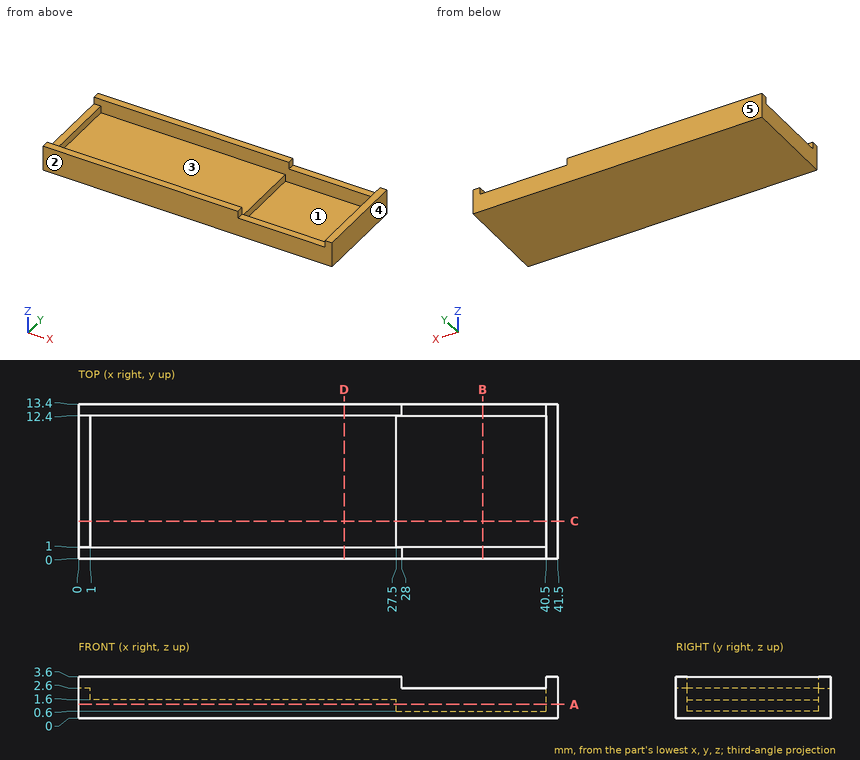
Input: dimensioned drawing with shaded views. Units: mm. Origin: part minimum x, y, z. A direction names the side the tool comes from. Round coordinates to 2 decimals unless told otherwise and drop trailing zeros. Order: outer loops, then holes, each group sorted by start corner. A loop starts at its lowest first (then second) coordinate and runs counter-clockwise, first axis right, second up.
1. Mould query, pull axis Y, two halves, no side actions, for the marked faces 3, 4 and 5. Classes: released by +Y, released by -Y, zero draft, split by the parting line, or undercut.
The answers:
face 3: undercut
face 4: zero draft
face 5: released by +Y
2. Material intervals for line 1 (Y direction, x = 5, z = 2.3); line 2 (X direction, y = 7, z = 1.95); line 3 (X direction, y = 7, z = 0.8), sorted ascending.
The answers:
line 1: y = 0 to 1, 12.4 to 13.4
line 2: x = 0 to 1, 40.5 to 41.5
line 3: x = 0 to 27.5, 40.5 to 41.5
3. Cut plane A-A, the plane z = 1.2. Output: boundary loops of the cut face in (x, y).
The answers:
outline: (0, 0) - (41.5, 0) - (41.5, 13.4) - (0, 13.4) - close; hole (27.5, 1) - (40.5, 1) - (40.5, 12.4) - (27.5, 12.4) - close
4. Set-up query: the marked faces 1 and 2. Return all of +Z, -Z, +X, -X, +Y, -Y with unobstructed straight access to the full face (end or side cutting, diameter ignored); none if empty.
The answers:
face 1: +Z
face 2: +Z, -Z, +X, -X, -Y
5. Cut plane B-B, the plane x = 35. Output: boundary loops of the cut face in (y, z), then the cut area to 3 significant figures.
The answers:
outline: (0, 0) - (13.4, 0) - (13.4, 2.6) - (12.4, 2.6) - (12.4, 0.6) - (1, 0.6) - (1, 2.6) - (0, 2.6) - close
area: 12.0 mm2
6. Pin query (flat end, axial travel): P1, Ø6, axis at x = 7.5, y = 5, coming from the +Z side; P2, Ø0.8, axis at x = 0.5, y = 9.5, coming from the +Z side; P3, Ø3.5, axis at x = 35, y = 7.5, coming from the +Z side. Return the tip coordinate at first contact, or that it passes through.
The answers:
P1: stops at z = 1.6
P2: stops at z = 2.6
P3: stops at z = 0.6
7. Cut plane C-C, the plane y = 3.25. Output: boundary loops of the cut face in (x, z), then the cut area to 3 significant figures.
The answers:
outline: (0, 0) - (41.5, 0) - (41.5, 3.6) - (40.5, 3.6) - (40.5, 0.6) - (27.5, 0.6) - (27.5, 1.6) - (1, 1.6) - (1, 2.6) - (0, 2.6) - close
area: 56.4 mm2
8. Cut plane D-D, the plane x = 23. Output: boundary loops of the cut face in (y, z).
The answers:
outline: (0, 0) - (13.4, 0) - (13.4, 3.6) - (12.4, 3.6) - (12.4, 1.6) - (1, 1.6) - (1, 3.6) - (0, 3.6) - close
